```python
from build123d import *

# Parameters (mm, degrees)
SKETCH2_R           = 15
SKETCH1_R           = 25
SKETCH3_R           = 15
BOSS_EXTRUDE1_DEPTH = 5
FILLET1_R           = 10
SKETCH4_R           = 1.75
CUT_EXTRUDE1_DEPTH  = 130
SKETCH5_R           = 4
CUT_EXTRUDE2_DEPTH  = 130
SKETCH6_R           = 22
BOSS_EXTRUDE2_DEPTH = 4
SKETCH7_R           = 17
BOSS_EXTRUDE3_DEPTH = 20
SKETCH15_W          = 8.431609766
SKETCH15_H          = 4
SKETCH15_W_2        = 8.578672696
SKETCH18_R          = 12.5
CUT_EXTRUDE5_DEPTH  = 20
SKETCH19_R          = 47.987160243
CUT_EXTRUDE6_DEPTH  = 44.301270362
SKETCH20_R          = 1.75
BOSS_EXTRUDE5_DEPTH = 4
CIRPATTERN3_COUNT   = 4
FILLET2_R           = 10
CHAMFER1_SIZE       = 0.5
SKETCH22_W          = 15
SKETCH22_H          = 8
BOSS_EXTRUDE6_DEPTH = 7.5
CUT_EXTRUDE7_DEPTH  = 0.75
CHAMFER2_SIZE       = 3
CHAMFER3_SIZE       = 0.5
CUT_EXTRUDE8_START  = -0.1
SKETCH24_R          = 41.017326151
SKETCH24_R_2        = 17
CUT_EXTRUDE8_DEPTH  = 0.1
SKETCH26_W          = 86.249785383
SKETCH26_H          = 35.556355766
CUT_EXTRUDE9_DEPTH  = 50
SKETCH27_R          = 10
BOSS_EXTRUDE7_DEPTH = 10
SKETCH28_R          = 37.5
BOSS_EXTRUDE8_DEPTH = 6
FILLET3_R           = 3


with BuildPart() as part:
    # Sketch2 → Loft1 section 0
    with BuildSketch(Plane.XY.offset(20)):
        Circle(SKETCH2_R)
    # Sketch1 → Loft1 section 1
    with BuildSketch(Plane.XY):
        Circle(SKETCH1_R)
    loft()

    # Sketch3 → Boss-Extrude1 (add)
    with BuildSketch(Plane.XY.offset(20)):
        Circle(SKETCH3_R)
    extrude(amount=BOSS_EXTRUDE1_DEPTH)

    # Fillet1
    fillet1_edges = [part.edges().sort_by_distance(p)[0] for p in [
        (-15, 0, 20),
    ]]
    fillet(fillet1_edges, radius=FILLET1_R)

    # Sketch4 → Cut-Extrude1 (cut)
    with BuildSketch(Plane(origin=(0, 0, 0), x_dir=(-1, 0, 0), z_dir=(0, 0, -1))):
        with Locations((0, 20)):
            Circle(SKETCH4_R)
        with Locations((-20, 0)):
            Circle(SKETCH4_R)
        with Locations((0, -20)):
            Circle(SKETCH4_R)
        with Locations((20, 0)):
            Circle(SKETCH4_R)
    extrude(amount=-CUT_EXTRUDE1_DEPTH, mode=Mode.SUBTRACT)

    # Sketch5 → Cut-Extrude2 (cut)
    with BuildSketch(Plane(origin=(0, 0, 3), x_dir=(-1, 0, 0), z_dir=(0, 0, -1))):
        with Locations((0, 20)):
            Circle(SKETCH5_R)
        with Locations((20, 0)):
            Circle(SKETCH5_R)
        with Locations((-20, 0)):
            Circle(SKETCH5_R)
        with Locations((0, -20)):
            Circle(SKETCH5_R)
    extrude(amount=-CUT_EXTRUDE2_DEPTH, mode=Mode.SUBTRACT)

    # Sketch6 → Boss-Extrude2 (add)
    with BuildSketch(Plane.XY.offset(25)):
        Circle(SKETCH6_R)
    extrude(amount=BOSS_EXTRUDE2_DEPTH)

    # Sketch7 → Boss-Extrude3 (add)
    with BuildSketch(Plane.XY.offset(29)):
        Circle(SKETCH7_R)
    extrude(amount=BOSS_EXTRUDE3_DEPTH)

    # Sketch15 → Cut-Revolve1 (revolve, cut)
    with BuildSketch(Plane(origin=(0, 0, 0), x_dir=(1, 0, 0), z_dir=(0, 1, 0))):
        with Locations((-17.215804883, -35)):
            Rectangle(SKETCH15_W, SKETCH15_H)
        with Locations((-17.289336348, -43)):
            Rectangle(SKETCH15_W_2, SKETCH15_H)
    revolve(axis=Axis((0, 0, 29), (0, 0, 1)), mode=Mode.SUBTRACT)

    # Sketch18 → Cut-Extrude5 (cut)
    with BuildSketch(Plane(origin=(0, 0, 0), x_dir=(-1, 0, 0), z_dir=(0, 0, -1))):
        Circle(SKETCH18_R)
    extrude(amount=-CUT_EXTRUDE5_DEPTH, mode=Mode.SUBTRACT)

    # Sketch19 → Cut-Extrude6 (cut, through all)
    with BuildSketch(Plane(origin=(0, 0, 25), x_dir=(-1, 0, 0), z_dir=(0, 0, -1))):
        Circle(SKETCH19_R)
    extrude(amount=CUT_EXTRUDE6_DEPTH, mode=Mode.SUBTRACT)

    # Sketch20 → Boss-Extrude5 (add)
    with BuildSketch(Plane(origin=(0, 0, 25), x_dir=(-1, 0, 0), z_dir=(0, 0, -1))):
        with BuildLine():
            Line((-4, 30), (-4, 21.633307653))
            ThreePointArc((-4, 21.633307653), (0, 22), (4, 21.633307653))
            Line((4, 21.633307653), (4, 30))
            ThreePointArc((4, 30), (0, 34), (-4, 30))
        make_face()
        with Locations((0, 30)):
            Circle(SKETCH20_R, mode=Mode.SUBTRACT)
    boss_extrude5 = extrude(amount=-BOSS_EXTRUDE5_DEPTH)

    # CirPattern3: Boss-Extrude5 ×4 about axis
    cirpattern3_axis = Axis((0, 0, 0), (0, 0, 1))
    for i in range(1, CIRPATTERN3_COUNT):
        add(boss_extrude5.rotate(cirpattern3_axis, i * 360 / CIRPATTERN3_COUNT))

    # Fillet2
    fillet2_edges = [part.edges().sort_by_distance(p)[0] for p in [
        (-4, 21.633307653, 27),
        (4, 21.633307653, 27),
        (-21.633307653, -4, 27),
        (-21.633307653, 4, 27),
        (4, -21.633307653, 27),
        (-4, -21.633307653, 27),
        (21.633307653, 4, 27),
        (21.633307653, -4, 27),
    ]]
    fillet(fillet2_edges, radius=FILLET2_R)

    # Chamfer1
    chamfer1_edges = [part.edges().sort_by_distance(p)[0] for p in [
        (-17, 0, 49),
        (-17, 0, 37),
        (-17, 0, 33),
        (-17, 0, 45),
        (-17, 0, 41),
    ]]
    chamfer(chamfer1_edges, length=CHAMFER1_SIZE)

    # Sketch22 → Boss-Extrude6 (add, symmetric)
    with BuildSketch(Plane(origin=(0, 0, 0), x_dir=(1, 0, 0), z_dir=(0, 1, 0))):
        with Locations((0, -53)):
            Rectangle(SKETCH22_W, SKETCH22_H)
    extrude(amount=BOSS_EXTRUDE6_DEPTH, both=True)

    # Sketch23 → Cut-Extrude7 (cut, symmetric)
    with BuildSketch(Plane(origin=(0, 0, 0), x_dir=(1, 0, 0), z_dir=(0, 1, 0))):
        with BuildLine():
            Line((7.5, -53.009618943), (7.5, -49))
            Line((7.5, -49), (-7.5, -49))
            Line((-7.5, -49), (-7.5, -53.009618943))
            ThreePointArc((-7.5, -53.009618943), (0, -51), (7.5, -53.009618943))
        make_face()
    extrude(amount=CUT_EXTRUDE7_DEPTH, both=True, mode=Mode.SUBTRACT)

    # Chamfer2
    chamfer2_edges = [part.edges().sort_by_distance(p)[0] for p in [
        (7.5, -7.5, 53),
        (-7.5, -7.5, 53),
        (7.5, 7.5, 53),
        (-7.5, 7.5, 53),
    ]]
    chamfer(chamfer2_edges, length=CHAMFER2_SIZE)

    # Chamfer3
    chamfer3_edges = [part.edges().sort_by_distance(p)[0] for p in [
        (-7.5, -2.625, 49),
        (7.5, -2.625, 49),
        (7.5, 2.625, 49),
        (7.5, 0, 57),
        (0, -7.5, 57),
        (0, -7.5, 49),
        (0, 7.5, 57),
        (-7.5, 0, 57),
        (-6, 6, 57),
        (-6, -6, 57),
        (6, 6, 57),
        (6, -6, 57),
        (0, 7.5, 49),
        (-7.5, 2.625, 49),
        (6, -6, 49),
        (6, 6, 49),
        (-6, -6, 49),
        (-6, 6, 49),
    ]]
    chamfer(chamfer3_edges, length=CHAMFER3_SIZE)

    # Sketch24 → Cut-Extrude8 (cut)
    with BuildSketch(Plane.XY.offset(29).offset(CUT_EXTRUDE8_START)):
        Circle(SKETCH24_R)
        with Locations(Location((0, 0, 0), (0, 0, 180))):
            Circle(SKETCH24_R_2, mode=Mode.SUBTRACT)
    extrude(amount=CUT_EXTRUDE8_DEPTH, mode=Mode.SUBTRACT)

    # Sketch26 → Cut-Extrude9 (cut, symmetric)
    with BuildSketch(Plane(origin=(0, 0, 0), x_dir=(1, 0, 0), z_dir=(0, 1, 0))):
        with Locations((1.892134232, -46.678177883)):
            Rectangle(SKETCH26_W, SKETCH26_H)
    extrude(amount=CUT_EXTRUDE9_DEPTH, both=True, mode=Mode.SUBTRACT)

    # Sketch27 → Boss-Extrude7 (add)
    with BuildSketch(Plane(origin=(0, 0, 25), x_dir=(-1, 0, 0), z_dir=(0, 0, -1))):
        Circle(SKETCH27_R)
    extrude(amount=BOSS_EXTRUDE7_DEPTH)

    # Sketch28 → Boss-Extrude8 (add)
    with BuildSketch(Plane(origin=(0, 0, 15), x_dir=(-1, 0, 0), z_dir=(0, 0, -1))):
        Circle(SKETCH28_R)
    extrude(amount=BOSS_EXTRUDE8_DEPTH)

    # Fillet3
    fillet3_edges = [part.edges().sort_by_distance(p)[0] for p in [
        (10, 0, 25),
        (10, 0, 15),
        (37.5, 0, 15),
        (37.5, 0, 9),
    ]]
    fillet(fillet3_edges, radius=FILLET3_R - 0.0001)  # a hair under: the kernel refuses the full size


solid = part.part
```
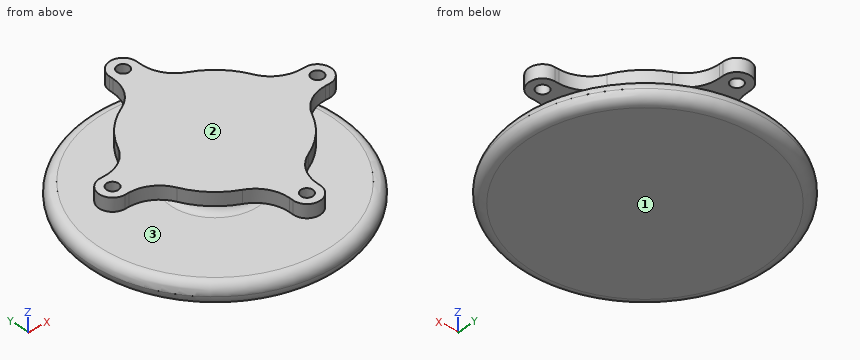
Can you work these out from the model? Positions are in its coordinate system, mm. Face numbers are marked on the shaded views. Coordinates: 2 decimals unless noted, no trailing zeros. Loops run counter-clockwise (first coordinate to the right, second up) from the corner with the lowest first, then second, coordinate; pieces in that order, holes last. Notation, with made-up numbers: (-22, 37.5) -> (-7, 37.5) arc R32 ccw to (-7, 75.5) -> close; hole circle Ø6 at (82, 20.25). An arc over 180 degrees is marked (long way). Answer as a JSON object with one key per item and string values.
1) Thinking about a two-plate mould opening in Z: for the marked faces 1, 2 and 3, which applies, pulls with the +Z half, pulls with the -Z half, needs draft (parallel to the pull), parting line crosses it, or undercut?
Results:
{"face 1": "pulls with the -Z half", "face 2": "pulls with the +Z half", "face 3": "undercut"}
2) If I drill on line 1 (X direction, y = 0, z = 25.85); line 2 (Z direction, x = -7, y = 11), over which ranges is the centre line in solid material (lowest first)?
Results:
{"line 1": "x = -34 to -31.75, -28.25 to 28.25, 31.75 to 34", "line 2": "z = 9 to 15, 25 to 28.9"}
3) Imagine slicing it at A-A (x = 0). Count the separate pieces of the cut face and the enclosed holes in it, then the cut area to 3 significant figures.
Results:
{"separate pieces": "3", "enclosed holes": "0", "area": "888 mm^2"}
4) Imagine slicing it at B-B (z = 21). Please give me the cut outline in (x, y), then the cut area to 3 significant figures.
Results:
{"outline": "circle Ø20 at (0, 0)", "area": "314 mm^2"}
5) Imagine slicing it at C-C (z = 13). Please give me the cut outline in (x, y).
Results:
{"outline": "circle Ø74.66 at (0, 0)"}
6) For P1, Ø0.6, axis at x = -29.5, z = 26.5, coming from the -Y side; P2, Ø3, axis at x = 12.5, y = -22.5, coming from the +Z side; P3, Ø0.6, axis at x = 29.5, z = 27.5, coming from the +Y side, each with a flat end and sliding along its axis, tell me the tip position at first contact or that it passes through.
Results:
{"P1": "stops at y = -4", "P2": "stops at z = 15", "P3": "stops at y = 4"}
